Here's how the part is built. I have some questions about the finished solid (model axes, mm). Face numbers are marked on the shaded views. A direction names the side the tool comes from. Round coordinates to 2 decimals unless told otherwise and drop trailing zeros. Loops run counter-clockwise (first coordinate to the right, second up) from the corner with the lowest first, then second, coordinate; pieces in that order, holes last. Notation, with made-up numbers: M 86,58.5 L 95,58.5 A10 ccw 95,65.5 Z; hole C 76.25,-27.75 d2. An arc over 180 degrees is marked long. Answer as a JSON object with one key per item and string values.
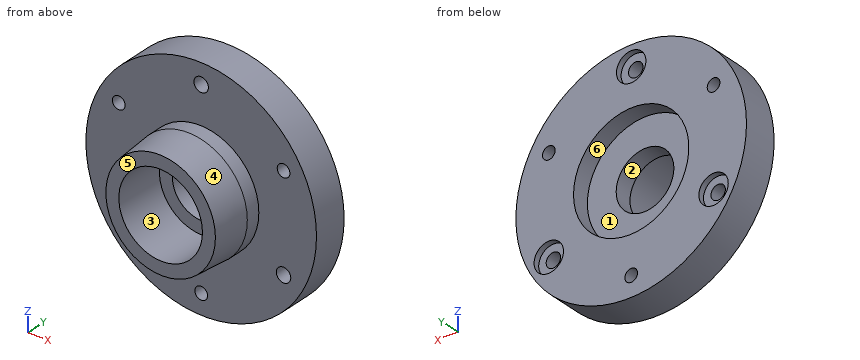
from build123d import *

# Parameters (mm, degrees)
F0_R            = 200
F0_R_2          = 100
F0_R_3          = 72.5
F0_R_4          = 50
F1_DEPTH        = 30
F2_DEPTH        = 118
F3_DEPTH        = 30
F5_D            = 25
F5_CBORE_D      = 51
F5_CBORE_DEPTH  = 10
F5_COPIES_COUNT = 3
F6_D            = 22
F6_COPIES_COUNT = 3
F7_SIZE2        = 63
F7_SIZE         = 5


# Not quite as in the source:
# - a pattern or mirror of a feature is missing from the dataset's text; its kind, count and spacing are read off the source's solid


with BuildPart() as f1:
    # F0 (on Front) → F1 (new body)
    with BuildSketch(Plane.XZ):
        Circle(F0_R)
        Circle(F0_R_2, mode=Mode.SUBTRACT)
        Circle(F0_R_2)
        Circle(F0_R_3, mode=Mode.SUBTRACT)
        Circle(F0_R_3)
        Circle(F0_R_4, mode=Mode.SUBTRACT)
    extrude(amount=F1_DEPTH)

    # F0 (on Front) → F2 (join)
    with BuildSketch(Plane.XZ):
        Circle(F0_R_2)
        Circle(F0_R_3, mode=Mode.SUBTRACT)
    extrude(amount=F2_DEPTH)

    # F0 (on Front) → F3 (join)
    with BuildSketch(Plane.XZ):
        Circle(F0_R)
        Circle(F0_R_2, mode=Mode.SUBTRACT)
    extrude(amount=-F3_DEPTH)

    # F5 (through all)
    with Locations(Plane(origin=(0, 30, 0), x_dir=(-1, 0, 0), z_dir=(0, 1, 0))):
        with Locations((0, 165)):
            f5 = CounterBoreHole(F5_D / 2, F5_CBORE_D / 2, F5_CBORE_DEPTH)

    # F5_copies: F5 ×3 about axis
    f5_copies_axis = Axis((0, 0, 0), (0, 1, 0))
    for i in range(1, F5_COPIES_COUNT):
        add(f5.rotate(f5_copies_axis, i * 360 / F5_COPIES_COUNT), mode=Mode.SUBTRACT)

    # F6 (through all)
    with Locations(Plane(origin=(0, 30, 0), x_dir=(-1, 0, 0), z_dir=(0, 1, 0))):
        with Locations((-142.8941916244, 82.5)):
            f6 = Hole(F6_D / 2)

    # F6_copies: F6 ×3 about axis
    f6_copies_axis = Axis((0, 0, 0), (0, 1, 0))
    for i in range(1, F6_COPIES_COUNT):
        add(f6.rotate(f6_copies_axis, i * 360 / F6_COPIES_COUNT), mode=Mode.SUBTRACT)

    # F7
    f7_edges = [f1.edges().sort_by_distance(p)[0] for p in [
        (-100, -118, 0),
    ]]
    f7_side = f1.faces().sort_by_distance((-97.171573, -118, 0))[0]
    chamfer(f7_edges, length=F7_SIZE, length2=F7_SIZE2, reference=f7_side)


solid = f1.part
Item 1: On a 3-axis mill with a long thin cutter (end or side, diameter ignored), from which of +Z, -Z, +X, -X, +Y, -Y can I reach the whole of each face in a straight line? I mean the marked faces 1, 2 and 3. Say none if no direction works.
Resolved:
{"face 1": "+Y", "face 2": "+Y, -Y", "face 3": "-Y"}
Item 2: I'm going to push flat-ended pins straight in: pin 1 Ø15 at (x, z) = (142.89, -82.5) entering from -Y (3 decimals); pin 2 Ø10 at (x, y) = (117, -7.5) entering from -Z; pin 3 Ø5 at (y, z) = (-66.5, 89) entering from +X; pin 4 Ø2 at (x, z) = (132.5, 22) entering from -Y. Where does each tip first touch, or does it pass through?
Resolved:
{"pin 1": "through", "pin 2": "z = -165.7", "pin 3": "x = 48.35", "pin 4": "y = -30"}
Item 3: If we mould it in two halves opening along Z, with no side actions, what happens to the marked faces 4, 5 and 6? For each: pulls with the +Z half, pulls with the -Z half, needs draft (parallel to the pull), parting line crosses it, or undercut.
Resolved:
{"face 4": "parting line crosses it", "face 5": "needs draft", "face 6": "undercut"}
Item 4: I want a section at D-D, the plane y = -49. Please give me the cut outline in (x, z).
Resolved:
{"outline": "C 0,0 d200; hole C 0,0 d145"}
Item 5: Please list where these lines run through material, in increasing order: probe 1 along Z at (x, y) = (0, -2); probe 2 along Z at (x, y) = (0, 13); probe 3 along X at (y, z) = (19.5, -90.5). Write a range as from..to.
Resolved:
{"probe 1": "-200..-176, -154..-50, 50..152.5, 177.5..200", "probe 2": "-200..-176, -154..-100, 100..152.5, 177.5..200", "probe 3": "-178.35..-152.5, -133.29..-42.54, 42.54..133.29, 152.5..178.35"}
Item 6: I want a section at B-B, the plane x = 0. State how many separate pieces and enclosed holes the cut face has, then the cut area to 3 significant figures.
Resolved:
{"separate pieces": "4", "enclosed holes": "0", "area": "16,400 mm²"}
Item 7: I want a section at A-A, the plane z = 0. Please give me the cut outline in (x, y), then the cut area to 3 significant figures.
Resolved:
{"outline": "M -200,-30 L -100,-30 L -100,-55 L -95,-118 L -72.5,-118 L -72.5,-30 L -50,-30 L -50,0 L -100,0 L -100,30 L -200,30 Z; M 50,-30 L 72.5,-30 L 72.5,-118 L 95,-118 L 100,-55 L 100,-30 L 200,-30 L 200,30 L 100,30 L 100,0 L 50,0 Z", "area": "19,500 mm²"}
Item 8: I want a section at C-C, the plane x = -143. Please give me the cut outline in (y, z).
Resolved:
{"outline": "M -30,-139.82 L 30,-139.82 L 30,-108 L 20,-108 L 20,-95 L -30,-95 Z; M -30,-70 L 20,-70 L 20,-57 L 30,-57 L 30,71.5 L -30,71.5 Z; M -30,93.5 L 30,93.5 L 30,139.82 L -30,139.82 Z"}
